Could you check a few things on this drawing? It's one solid part, dimensions in mm from its lowest x, y, z. A direction names the side the tool comes from. Coordinates: 2 decimals unless noted, no trailing zeros. Order: outer loops, then holes, each group sorted by start corner. A loop starts at its lowest first (then second) coordinate and runs counter-clockwise, first axis right, second up. Notation, with made-up numbers: (33.25, 31.25) - (78.25, 31.25) arc R12 cw to (78.25, 38.25) - close; hole circle Ø10 at (-8.75, 45.5). An arc over 180 degrees is marked (long way). Return JSON: item names as keys, results as strings. Group by question number.
1) If I drill on line 1 along Z through (x, y) = (41, 2) (3 decimals); line 2 along Y through (x, z) = (9.35, 29.75); line 3 along X through (y, z) = (40, 4.5), over which ranges is the centre line in solid material (lowest first)?
2) Imagine slicing it at C-C (x = 40). Write out the boundary of the cut face in (y, z) (3 decimals), and give its area (3 significant figures).
3) Imagine slicing it at A-A (y = 12.7). Write out the boundary of the cut face in (x, z) (3 decimals).
4) Imagine slicing it at D-D (y = 5). Write out the boundary of the cut face in (x, z) (3 decimals), and give its area (3 significant figures).
5) For pin 1 Ø1 at (x, z) = (13.5, 24) entering from +Y; pin 2 Ø8 at (x, z) = (31, 8) entering from -Y, each with a flat end and sliding along its axis, tell me the tip position at first contact or that it passes through.
6) Imagine slicing it at B-B (z = 22). Write out the boundary of the cut face in (x, y), and give its area (3 significant figures).
7) If we mould it in two halves opening along X, with no side actions, what happens to the marked faces 4, 5, 6 and 7? For each: pulls with the +X half, pulls with the -X half, needs draft (parallel to the pull), parting line crosses it, or undercut.
8) Which directions (+Z, -Z, +X, -X, +Y, -Y) give clear straight access to the entire face, cutting with the end or side of a thin tool? Please do the marked faces 1, 2 and 3.
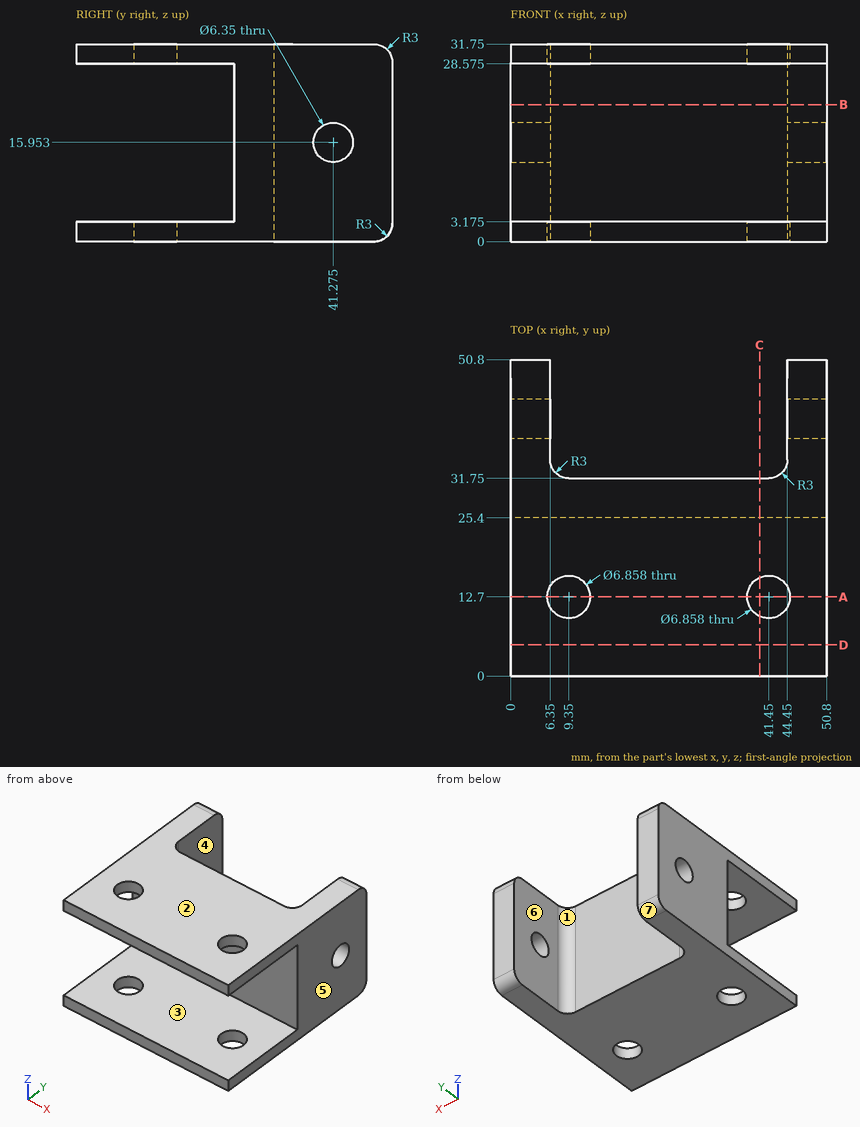
Calculated:
{
 "1": {"line 1": "0 to 3.175, 28.575 to 31.75", "line 2": "0 to 9.27, 16.13 to 31.75", "line 3": "0 to 6.35, 44.45 to 50.8"},
 "2": {"outline": "(0, 0) - (9.593, 0) - (9.593, 3.175) - (0, 3.175) - close; (0, 28.575) - (9.593, 28.575) - (9.593, 31.75) - (0, 31.75) - close; (15.807, 0) - (31.75, 0) - (31.75, 31.75) - (15.807, 31.75) - (15.807, 28.575) - (25.4, 28.575) - (25.4, 3.175) - (15.807, 3.175) - close", "area": "323 mm2"},
 "3": {"outline": "(0, 0) - (5.921, 0) - (5.921, 3.175) - (0, 3.175) - close; (0, 28.575) - (5.921, 28.575) - (5.921, 31.75) - (0, 31.75) - close; (12.779, 0) - (38.021, 0) - (38.021, 3.175) - (12.779, 3.175) - close; (12.779, 28.575) - (38.021, 28.575) - (38.021, 31.75) - (12.779, 31.75) - close; (44.879, 0) - (50.8, 0) - (50.8, 3.175) - (44.879, 3.175) - close; (44.879, 28.575) - (50.8, 28.575) - (50.8, 31.75) - (44.879, 31.75) - close"},
 "4": {"outline": "(0, 0) - (50.8, 0) - (50.8, 3.175) - (0, 3.175) - close; (0, 28.575) - (50.8, 28.575) - (50.8, 31.75) - (0, 31.75) - close", "area": "323 mm2"},
 "5": {"pin 1": "y = 31.75", "pin 2": "y = 25.4"},
 "6": {"outline": "(0, 25.4) - (50.8, 25.4) - (50.8, 50.8) - (44.45, 50.8) - (44.45, 34.75) arc R3 cw to (41.45, 31.75) - (9.35, 31.75) arc R3 cw to (6.35, 34.75) - (6.35, 50.8) - (0, 50.8) - close", "area": "568 mm2"},
 "7": {"face 4": "undercut", "face 5": "pulls with the +X half", "face 6": "undercut", "face 7": "needs draft"},
 "8": {"face 1": "+Z, -Z, +Y", "face 2": "+Z, +X, -X, +Y, -Y", "face 3": "+X, -X, -Y"}
}
